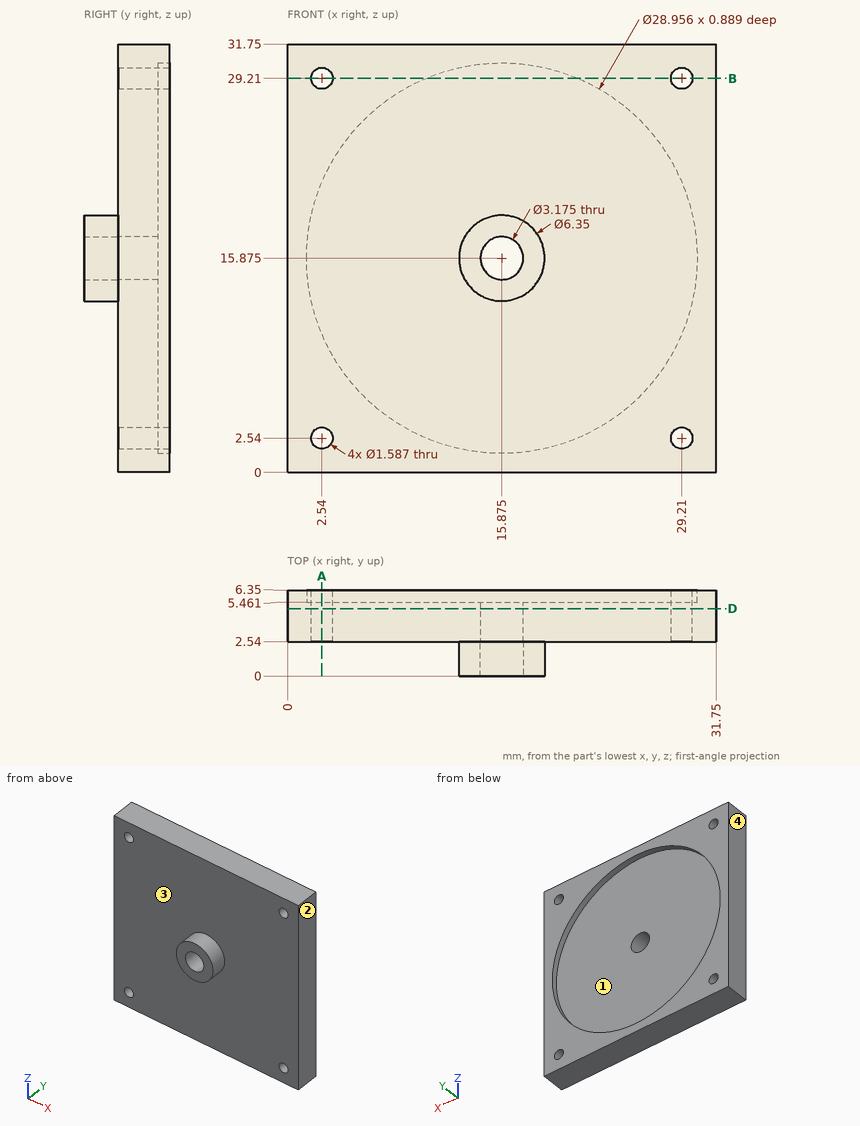
Job drawing, mm, ordinate dimensions from the low corner. One solid piece. Give positions to 0.01 mm unless a question says otherwise; leave off trailing zeros. Write each loop counter-clockwise with the first axis right and the second up, starting at its lowest first coordinate (ties: lowest second). Pieces come first, ordered by that corner, then holes. Notation, with made-up numbers: (11, 63.5) - (45, 63.5) arc R24 ccw to (45, 102.5) - close; hole circle Ø9 at (25, 17). An arc over 180 degrees is marked (long way). Use one line per item in the form item = value. Start each with the question number.
1. Drop flat-ended pins along their axis: pin 1 Ø2 at (y, z) = (1, 17.5) entering from +X; pin 2 Ø4 at (x, z) = (7, 24.5) entering from -Y; pin 3 Ø8.5 at (x, z) = (14, 20) entering from +Y. Give the stop position or say it passes through.
2. Band-saw the part on D-D on y = 5. Count the separate pieces of the cut face and the enclosed holes in it, plus the area to 3 significant figures.
3. Probe line 1 (Z direction, x = 29.21, y = 4.4); line 2 (Y direction, x = 13, z = 6); line 3 (Y direction, x = 29, z = 26). List the from-to ranges inside material, lowest first. Write a range as [from, to].
4. Band-saw the part on A-A on x = 2.54. Write the cut outline in (y, z).
5. Two-plate mould, pull along X, no slides. Class the marked faces 1, 2, 3 and 4: released by +X, released by -X, zero draft, split by the parting line, or undercut.
6. Band-saw the part on B-B on z = 29.21. Write the cut outline in (x, y).
Conclusion:
q1.pin_1 = 18.99
q1.pin_2 = 2.54
q1.pin_3 = 5.46
q2.separate_pieces = 1
q2.enclosed_holes = 5
q2.area = 992 mm²
q3.line_1 = [0, 1.75], [3.33, 28.42], [30, 31.75]
q3.line_2 = [2.54, 5.46]
q3.line_3 = [2.54, 6.35]
q4.outline = (2.54, 0) - (6.35, 0) - (6.35, 1.75) - (2.54, 1.75) - close; (2.54, 3.33) - (6.35, 3.33) - (6.35, 10.24) - (5.46, 10.24) - (5.46, 21.51) - (6.35, 21.51) - (6.35, 28.42) - (2.54, 28.42) - close; (2.54, 30) - (6.35, 30) - (6.35, 31.75) - (2.54, 31.75) - close
q5.face_1 = undercut
q5.face_2 = released by +X
q5.face_3 = zero draft
q5.face_4 = released by -X
q6.outline = (0, 2.54) - (1.75, 2.54) - (1.75, 6.35) - (0, 6.35) - close; (3.33, 2.54) - (28.42, 2.54) - (28.42, 6.35) - (21.51, 6.35) - (21.51, 5.46) - (10.24, 5.46) - (10.24, 6.35) - (3.33, 6.35) - close; (30, 2.54) - (31.75, 2.54) - (31.75, 6.35) - (30, 6.35) - close
